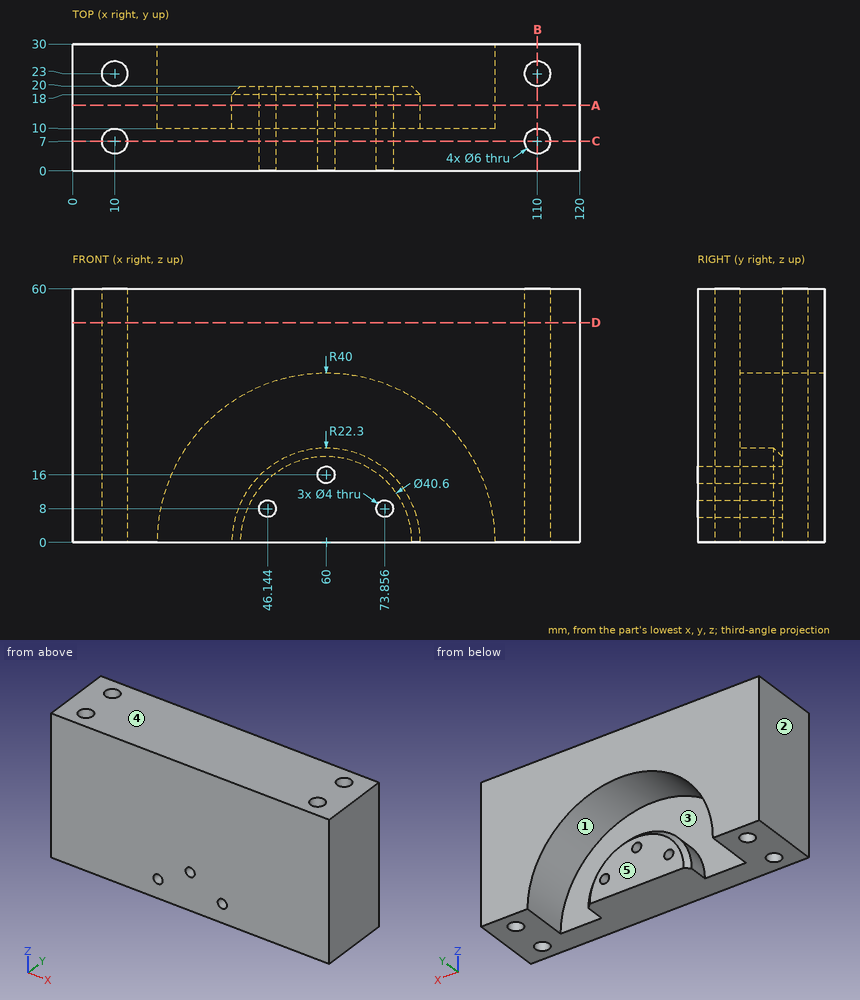
Study the drawing (mm; zero at the part's minimum x, y, z) and answer. A direction names the side the tool comes from. Coordinates: 2 decimals unless noted, no trailing zeros. Order: outer loops, then holes, each group sorted by start corner. A loop starts at its lowest first (then second) coordinate and runs counter-clockwise, first axis right, second up. Notation, with made-up numbers: M 56.5,-30 L 114.5,-30 A11 cw 114.5,-18 Z; hole C 70.25,22.5 d2. An arc over 180 degrees is marked long. Use CSV: the item, a comma, the result in double quotes.
Q1. Section A-A (y = 15.5) is taken. Determine the outline of the cut face in (x, z).
Here are the results:
outline,"M 0,0 L 20,0 A40 cw 100,0 L 120,0 L 120,60 L 0,60 Z; M 37.7,0 L 82.3,0 A22.3 ccw Z; hole C 46.14,8 d4; hole C 60,16 d4; hole C 73.86,8 d4"
Q2. Section B-B (x = 110) is taken. Determine the outline of the cut face in (y, z), then the cut area to 3 significant figures.
Here are the results:
outline,"M 0,0 L 4,0 L 4,60 L 0,60 Z; M 10,0 L 20,0 L 20,60 L 10,60 Z; M 26,0 L 30,0 L 30,60 L 26,60 Z"
area,"1,080 mm2"
Q3. Section D-D (z = 52) is taken. Determine the outline of the cut face in (x, y).
Here are the results:
outline,"M 0,0 L 120,0 L 120,30 L 0,30 Z; hole C 10,7 d6; hole C 10,23 d6; hole C 110,7 d6; hole C 110,23 d6"
Q4. Section C-C (y = 7) is taken. Determine the outline of the cut face in (x, z), then the cut area to 3 significant figures.
Here are the results:
outline,"M 0,0 L 7,0 L 7,60 L 0,60 Z; M 13,0 L 107,0 L 107,60 L 13,60 Z; M 113,0 L 120,0 L 120,60 L 113,60 Z; hole C 46.14,8 d4; hole C 60,16 d4; hole C 73.86,8 d4"
area,"6,440 mm2"
Q5. Given pin 1 Ø3 at (x, z) = (34.5, 14) entering from +Y; pin 2 Ø6 at (x, z) = (69.5, 7) entering from +Y; pin 3 Ø9.5 at (x, y) = (10, 7) entering from +Z; pin 4 Ø2 at (x, y) = (30, 22.5) entering from -Z, each flat-ended and moving along its own axis, determine where each tip first touches the part or whether it passes through.
Here are the results:
pin 1,"y = 10"
pin 2,"y = 20"
pin 3,"z = 60"
pin 4,"z = 25.28"
Q6. Straight lines are drawn through the part: L1, parallel to Y at x = 10, z = 45; L2, parallel to Y at x = 8.5, z = 34.5; L3, parallel to X at y = 23.75, z = 56 (1 decimal). For each, find the intervals that lie inside material, in ascending order.
Here are the results:
L1,"0 to 4, 10 to 20, 26 to 30"
L2,"0 to 4.4, 9.6 to 20.4, 25.6 to 30"
L3,"0 to 7.1, 12.9 to 107.1, 112.9 to 120"
Q7. Determine the mould class of the marked faces 3, 4 and 5 for opening direction Z: pulls with the +Z half, pulls with the -Z half, needs draft (parallel to the pull), parting line crosses it, or undercut.
Here are the results:
face 3,"undercut"
face 4,"pulls with the +Z half"
face 5,"needs draft"
Q8. A tool of negligible diameter and unlimited length cuts with its end or side. For the marked faces 1 and 2, from which of +Z, -Z, +X, -X, +Y, -Y can it reach the whole face along a straight path? Write none if from no direction.
Here are the results:
face 1,"+Y"
face 2,"+Z, -Z, -X, +Y, -Y"
